Source: CAD feature listing. Evaluate the final solid. Frame: model axes, mm. Face numbers are marked on the shaded views. A direction names the side the tool comes from. Coordinates: 2 decimals unless noted, no trailing zeros. Loops run counter-clockwise (first coordinate to the right, second up) from the corner with the lowest first, then second, coordinate; pieces in that order, holes last.
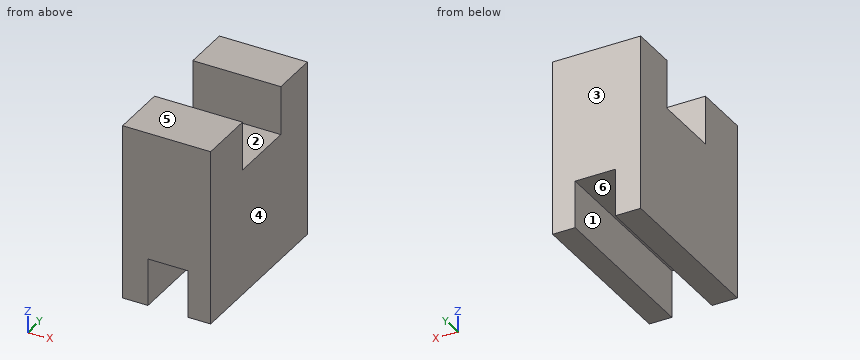
```python
from build123d import *

# Parameters (mm, degrees)
F1_DEPTH = 12.7
F4_W     = 5.7911989279
F4_H     = 6.8580000661
F5_DEPTH = 12.7
F6_DEPTH = 25.4


# Not quite as in the source:
# - a feature of the source that left no trace in its solid (it failed there, or was rolled back) is left out


with BuildPart() as f1:
    # F0 (on Right) → F1 (new body)
    with BuildSketch(Plane.YZ):
        Polygon((12.4962570041, 25.4), (12.4962570041, 0), (37.2171103641, 0), (37.2171103641, 25.4), (30.4256705266, 25.4), (30.4256705266, 18.3368995143), (20.6459868013, 18.3368995143), (20.6459868013, 25.4), align=None)
    extrude(amount=F1_DEPTH)

    # F4 (on Front) → F5 (cut)
    with BuildSketch(Plane.XZ):
        with Locations((6.553200772, 3.4290000331)):
            Rectangle(F4_W, F4_H)
    extrude(amount=-F5_DEPTH, mode=Mode.SUBTRACT)

    # F6 (cut): a face of the model
    f6_faces = [f1.faces().sort_by_distance(p)[0] for p in [
        (6.553200772, 12.7, 3.4290000331),
    ]]
    extrude(f6_faces, amount=-F6_DEPTH, mode=Mode.SUBTRACT)


solid = f1.part
```
Q1. Reachability of the marked faces 1, 2 and 3 from +Z, -Z, +X, -X, +Y, -Y: full face, straight path, thin tool, end or side. Return the list, or none.
Q2. Section query C-C on x = 1.5. Return the cut outline in (y, z).
Q3. Draft query along X for the marked faces 4, 5 and 6. Return one class per face: released by +X, released by -X, zero draft, split by the parting line, or undercut.
Q4. Material intervals for line 1 along X through (y, z) = (25, 3.5); line 2 along Y through (x, z) = (8.5, 24.25); line 3 along Z through (x, y) = (2.75, 29.75), sorted ascending.
Q5. Section query B-B on y = 22. Return the cut outline in (x, z).
Q6. Section query D-D on z = 19. Return the cut outline in (x, y).
Q7. First-contact query: pin 1 Ø3 at (x, y) = (6, 22) entering from -Z; pin 2 Ø2 at (x, y) = (4, 23) entering from +Z. Flat tips, straight axial feed; report the tip coordinate or a pass-through.
Q8. Section query A-A on z = 5.25. Return the cut outline in (x, y), then the cut area to 3 significant figures.
Resolved:
1. face 1: -Z, +Y, -Y
1. face 2: +Z, +X, -X
1. face 3: +Z, -Z, +X, -X, +Y
2. outline: (12.5, 0) - (37.22, 0) - (37.22, 25.4) - (30.43, 25.4) - (30.43, 18.34) - (20.65, 18.34) - (20.65, 25.4) - (12.5, 25.4) - close
3. face 4: released by +X
3. face 5: zero draft
3. face 6: undercut
4. line 1: x = 0 to 3.66, 9.45 to 12.7
4. line 2: y = 12.5 to 20.65, 30.43 to 37.22
4. line 3: z = 0 to 18.34
5. outline: (0, 0) - (3.66, 0) - (3.66, 6.86) - (9.45, 6.86) - (9.45, 0) - (12.7, 0) - (12.7, 18.34) - (0, 18.34) - close
6. outline: (0, 12.5) - (12.7, 12.5) - (12.7, 20.65) - (0, 20.65) - close; (0, 30.43) - (12.7, 30.43) - (12.7, 37.22) - (0, 37.22) - close
7. pin 1: stops at z = 6.86
7. pin 2: stops at z = 18.34
8. outline: (0, 12.5) - (3.66, 12.5) - (3.66, 37.22) - (0, 37.22) - close; (9.45, 12.5) - (12.7, 12.5) - (12.7, 37.22) - (9.45, 37.22) - close
8. area: 171 mm2
